Could you check a few things on this model? Use its own coordinates, in mm. Face numbers are marked on the shaded views. A direction names the side the tool comes from. Give positions to 0.01 mm unless a question says otherwise; leave off trailing zeros. Loops run counter-clockwise (first coordinate to the right, second up) from the corner with the lowest first, then second, coordinate; pieces in that order, holes last. Notation, with made-up numbers: (21.25, -29.5) - (48.25, -29.5) arc R14 cw to (48.25, -24.5) - close; hole circle Ø3 at (61, 24). An arc over 180 degrees is marked (long way). One line per item, written item: value. Start each with the question number.
Q1. I want a section at B-B (z = 11). Please give me the cut outline in (x, y) (3 decimals), then the cut area to 3 significant figures.
Q2. If I drill on line 1 (Y direction, x = -16.35, z = 11) (3 decimals); line 2 (Z direction, x = -5, y = 16); line 3 (X direction, y = -2.5, z = 12.25), over which ranges is the centre line in solid material (lowest first)? Write a range as from..to.
Q3. I'm going to push flat-ended pins straight in: P1, Ø18, axis at x = -6, y = 6, coming from the +Z side; P2, Ø0.8, axis at x = -17, z = 12.5, coming from the -Y side. Where does each tip first touch, or does it pass through?
Q4. For the marked faces 1 and 2, which set-ups out of +Z, -Z, +X, -X, +Y, -Y let a thin tool reach every point of the face, with its end or its side?
Q5. I want a section at A-A (y = 0). Please give me the cut outline in (x, z) (3 decimals).
Q6. I want a section at C-C (x = -11). Please give me the cut outline in (y, z), then the cut area to 3 significant figures.
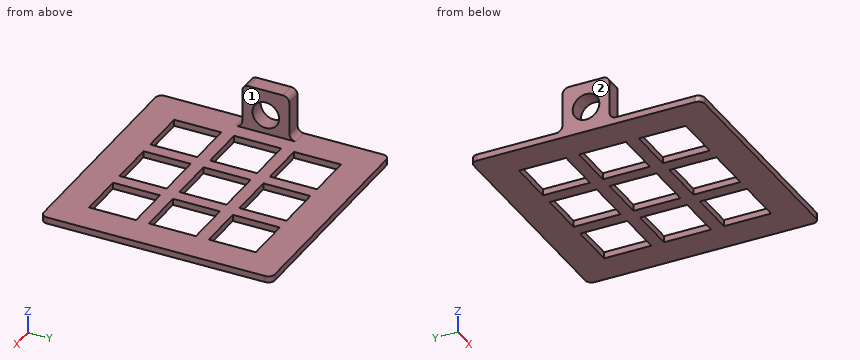
```python
from build123d import *

# Parameters (mm, degrees)
SKETCH1_W                  = 36
SKETCH1_H                  = 36
BOSS_EXTRUDE1_DEPTH        = 10
SKETCH2_W                  = 7.333333333
SKETCH2_H                  = 7.333333333
SKETCH2_H_2                = 7.333333334
SKETCH2_W_2                = 7.333333334
CUT_EXTRUDE1_DEPTH         = 28.349588662
SKETCH6_W                  = 36
SKETCH6_H                  = 36
CUT_EXTRUDE3_DEPTH         = 7
SKETCH9_W                  = 31.197314423
SKETCH9_H                  = 36.13311488
CUT_EXTRUDE5_DEPTH         = 2
SKETCH13_W                 = 5
SKETCH13_H                 = 36
BOSS_EXTRUDE2_DEPTH        = 10
F_4_1_4_1_DIAMETER_SLOT1_D = 4.15
CUT_EXTRUDE6_DEPTH         = 42.048751504
FILLET1_R                  = 1
CUT_EXTRUDE7_START         = -7
SKETCH17_W                 = 2.5
SKETCH17_H                 = 7.333333334
CUT_EXTRUDE7_DEPTH         = 7
FILLET2_R                  = 1


with BuildPart() as part:
    # Sketch1 → Boss-Extrude1 (new body)
    with BuildSketch(Plane.XY):
        Rectangle(SKETCH1_W, SKETCH1_H)
    extrude(amount=BOSS_EXTRUDE1_DEPTH)

    # Sketch2 → Cut-Extrude1 (cut, through all)
    with BuildSketch(Plane.XY.offset(10)):
        with Locations((-9.333333334, 9.333333334)):
            Rectangle(SKETCH2_W, SKETCH2_H)
        with Locations((-9.333333334, 0)):
            Rectangle(SKETCH2_W, SKETCH2_H_2)
        with Locations((0, 9.333333334)):
            Rectangle(SKETCH2_W_2, SKETCH2_H)
        Rectangle(SKETCH2_W_2, SKETCH2_H_2)
        with Locations((9.333333334, 9.333333334)):
            Rectangle(SKETCH2_W, SKETCH2_H)
        with Locations((9.333333334, 0)):
            Rectangle(SKETCH2_W, SKETCH2_H_2)
        with Locations((9.333333334, -9.333333334)):
            Rectangle(SKETCH2_W, SKETCH2_H)
        with Locations((0, -9.333333334)):
            Rectangle(SKETCH2_W_2, SKETCH2_H)
        with Locations((-9.333333334, -9.333333334)):
            Rectangle(SKETCH2_W, SKETCH2_H)
    extrude(amount=-CUT_EXTRUDE1_DEPTH, mode=Mode.SUBTRACT)

    # Sketch6 → Cut-Extrude3 (cut)
    with BuildSketch(Plane(origin=(0, 0, 0), x_dir=(-1, 0, 0), z_dir=(0, 0, -1))):
        Rectangle(SKETCH6_W, SKETCH6_H)
    extrude(amount=-CUT_EXTRUDE3_DEPTH, mode=Mode.SUBTRACT)

    # Sketch9 → Cut-Extrude5 (cut)
    with BuildSketch(Plane.XY.offset(10)):
        with Locations((2.598657212, 0.06655744)):
            Rectangle(SKETCH9_W, SKETCH9_H)
    extrude(amount=-CUT_EXTRUDE5_DEPTH, mode=Mode.SUBTRACT)

    # Sketch13 → Boss-Extrude2 (add)
    with BuildSketch(Plane.XY.offset(10)):
        with Locations((-15.5, 0)):
            Rectangle(SKETCH13_W, SKETCH13_H)
    extrude(amount=BOSS_EXTRUDE2_DEPTH)

    # Ø4.1 (4.1) Diameter Slot1 (through all)
    with Locations(Plane(origin=(-13, 0, 0), x_dir=(0, 0, -1), z_dir=(1, 0, 0))):
        with Locations((-11, 0)):
            Hole(F_4_1_4_1_DIAMETER_SLOT1_D / 2)

    # Sketch16 → Cut-Extrude6 (cut, through all)
    with BuildSketch(Plane(origin=(-13, 0, 0), x_dir=(0, 0, -1), z_dir=(1, 0, 0))):
        Polygon((-8, -18), (-8, -3.666666667), (-15, -3.666666667), (-15, 3.666666667), (-8, 3.666666667), (-8, 18), (-20, 18), (-20, -18), align=None)
    extrude(amount=-CUT_EXTRUDE6_DEPTH, mode=Mode.SUBTRACT)

    # Fillet1
    fillet1_edges = [part.edges().sort_by_distance(p)[0] for p in [
        (18, -18, 7.5),
        (18, 18, 7.5),
        (-18, -18, 7.5),
        (-18, 18, 7.5),
        (-15.5, 3.666666667, 15),
        (-15.5, -3.666666667, 15),
    ]]
    fillet(fillet1_edges, radius=FILLET1_R)

    # Sketch17 → Cut-Extrude7 (cut)
    with BuildSketch(Plane.XY.offset(15).offset(CUT_EXTRUDE7_START)):
        with Locations((-14.25, 0)):
            Rectangle(SKETCH17_W, SKETCH17_H)
    extrude(amount=CUT_EXTRUDE7_DEPTH, mode=Mode.SUBTRACT)

    # Fillet2
    fillet2_edges = [part.edges().sort_by_distance(p)[0] for p in [
        (-16.75, 3.666666667, 8),
        (-16.75, -3.666666667, 8),
    ]]
    fillet(fillet2_edges, radius=FILLET2_R)


solid = part.part
```
Worked answers:
1. outline: (-18, -3.667) - (-15.5, -3.667) - (-15.5, -2.075) - (-18, -2.075) - close; (-18, 2.075) - (-15.5, 2.075) - (-15.5, 3.667) - (-18, 3.667) - close
1. area: 7.96 mm²
2. line 1: y = -3.667..-2.075, 2.075..3.667
2. line 2: z = 7..8
2. line 3: x = -18..-15.5
3. P1: stops at z = 8
3. P2: stops at y = -3.67
4. face 1: +Z, +X, +Y, -Y
4. face 2: +Z, -Z, -X, +Y, -Y
5. outline: (-18, 7) - (-13, 7) - (-13, 8) - (-15.5, 8) - (-15.5, 8.925) - (-18, 8.925) - close; (-18, 13.075) - (-15.5, 13.075) - (-15.5, 15) - (-18, 15) - close; (-5.667, 7) - (-3.667, 7) - (-3.667, 8) - (-5.667, 8) - close; (3.667, 7) - (5.667, 7) - (5.667, 8) - (3.667, 8) - close; (13, 7) - (18, 7) - (18, 8) - (13, 8) - close
6. outline: (-18, 7) - (-13, 7) - (-13, 8) - (-18, 8) - close; (-5.67, 7) - (-3.67, 7) - (-3.67, 8) - (-5.67, 8) - close; (3.67, 7) - (5.67, 7) - (5.67, 8) - (3.67, 8) - close; (13, 7) - (18, 7) - (18, 8) - (13, 8) - close
6. area: 14.0 mm²
